Work out the finished part from the listing and answer in its coordinate system (mm). A direction names the side the tool comes from. Give positions to 0.01 mm unless a question says otherwise; leave off trailing zeros. Write each loop counter-clockwise with the first axis right and the second up, starting at its lowest first coordinate (ties: lowest second). Pieces come first, ordered by that corner, then holes. Notation, with made-up numbers: (-18.75, 11) - (-10.75, 11) arc R16 cw to (-10.75, 29) - close; hole circle Ø10 at (-12, 18.5). An arc over 180 degrees is marked (long way). Write item = value, one per line.
from build123d import *

# Parameters (mm, degrees)
F1_DEPTH = 228.6


with BuildPart() as f1:
    # F0 (on Top) → F1 (new body)
    with BuildSketch(Plane.XY):
        with BuildLine():
            ThreePointArc((-12.7, -11.1125), (-12.235032, -12.235032), (-11.1125, -12.7))
            Line((-11.1125, -12.7), (-3.3655, -12.7))
            Line((-3.3655, -12.7), (-3.3655, -9.525))
            Line((-3.3655, -9.525), (-9.525, -9.525))
            Line((-9.525, -9.525), (-9.525, -1.315128))
            Line((-9.525, -1.315128), (-2.245064, 5.964808))
            ThreePointArc((-2.245064, 5.964808), (0, 6.894744), (2.245064, 5.964808))
            Line((2.245064, 5.964808), (9.525, -1.315128))
            Line((9.525, -1.315128), (9.525, -9.525))
            Line((9.525, -9.525), (3.3655, -9.525))
            Line((3.3655, -9.525), (3.3655, -12.7))
            Line((3.3655, -12.7), (11.1125, -12.7))
            ThreePointArc((11.1125, -12.7), (12.235032, -12.235032), (12.7, -11.1125))
            Line((12.7, -11.1125), (12.7, -2.630256))
            ThreePointArc((12.7, -2.630256), (12.216635, -0.200216), (10.840128, 1.859872))
            Line((10.840128, 1.859872), (4.490128, 8.209872))
            ThreePointArc((4.490128, 8.209872), (0, 10.069744), (-4.490128, 8.209872))
            Line((-4.490128, 8.209872), (-10.840128, 1.859872))
            ThreePointArc((-10.840128, 1.859872), (-12.216635, -0.200216), (-12.7, -2.630256))
            Line((-12.7, -2.630256), (-12.7, -11.1125))
        make_face()
    extrude(amount=F1_DEPTH)


solid = f1.part
1. Given pin 1 (7 mm diameter, centred on x = 6, z = 81, fed in from +Y); pin 2 (1.8 mm diameter, centred on x = -5.5, z = 79.5, fed in from +Y); pin 3 (1 mm diameter, centred on x = -2, y = -10.5, fed in from -Z); pin 4 (12 mm diameter, centred on y = 4, z = 76.5, fed in from -X), each flat-ended and moving along its own axis, determine where each tip first touches the part or whether it passes through.
Solution:
pin_1 = 9.56
pin_2 = 8.1
pin_3 = through
pin_4 = -12.67
2. For a pull along X with two mould halves and no side action, classify faces 1 (the flat face through (7, -12.7, 113)), 2 (the flat face through (-6, -9.525, 113)), 3 (the flat face through (-7.6, 5.1, 112.7)) as pulls with the +X half, pulls with the -X half, needs draft (parallel to the pull), parting line crosses it, or undercut.
Solution:
face_1 = needs draft
face_2 = undercut
face_3 = pulls with the -X half
3. Find section A-A, the plane y = -4.5. Give the vertices of the cut face in (x, z) (3 decimals), then the cut area to 3 significant figures.
Solution:
outline = (-12.7, 0) - (-9.525, 0) - (-9.525, 228.6) - (-12.7, 228.6) - close; (9.525, 0) - (12.7, 0) - (12.7, 228.6) - (9.525, 228.6) - close
area = 1,450 mm^2
4. A tool of negligible diameter and unlimited length cuts with its end or side. For faces 4 (the flat face through (-5.94, 2.27, 112.7)), 5 (the cylindrical face through (-12.203, -0.168, 112.7)), from which of +Z, -Z, +X, -X, +Y, -Y can it reach the whole face along a straight path? Write none if from no direction.
Solution:
face_4 = +Z, -Z
face_5 = +Z, -Z, -X, +Y
5. Find section C-C, the plane x = 0. Give the vertices of the cut face in (y, z).
Solution:
outline = (6.89, 0) - (10.07, 0) - (10.07, 228.6) - (6.89, 228.6) - close
6. Straight lines are drawn through the part: line 1 (X direction, y = -10, z = 135.5); line 2 (X direction, y = -6, z = 146) (3 decimals); line 3 (Y direction, x = 0, z = 34.5). For each, find the intervals that lie inside material, in ascending order.
Solution:
line_1 = -12.7 to -3.37, 3.37 to 12.7
line_2 = -12.7 to -9.525, 9.525 to 12.7
line_3 = 6.89 to 10.07
